Drawing for the job (mm, zero at the part's lowest x, y, z). A direction names the side the tool comes from. Coordinates: 2 decimals unless noted, no trailing zeros. Write each loop counter-clockwise with the first axis right and the second up, starting at its lowest first coordinate (ties: lowest second). Pieces come first, ordered by that corner, then holes. Notation, with made-up numbers: (-11, 83.5) - (32, 83.5) arc R20 cw to (32, 88.5) - close; hole circle Ø1 at (43, -1). An arc over 180 degrees is marked (long way). Write each question's results on one line, items separated by ' | '.
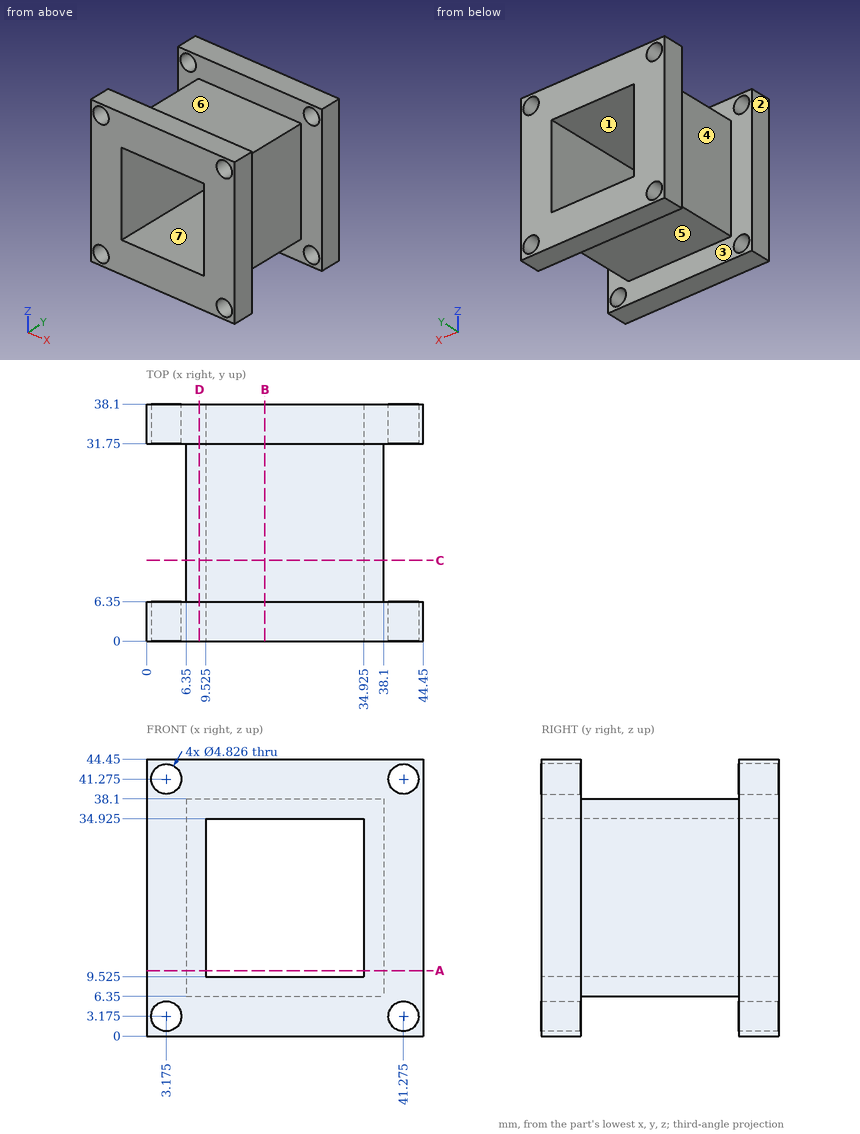
(1) Saw through at C-C on y = 13. Write the cut outline in (x, z) (3 decimals), then the cut area to 3 significant figures.
Return value:
outline: (6.35, 6.35) - (38.1, 6.35) - (38.1, 38.1) - (6.35, 38.1) - close; hole (9.525, 9.525) - (34.925, 9.525) - (34.925, 34.925) - (9.525, 34.925) - close | area: 363 mm^2
(2) Two-plate mould, pull along X, no slides. Class the marked faces 1, 2 and 3: released by +X, released by -X, zero draft, split by the parting line, or undercut.
Return value:
face 1: undercut | face 2: released by -X | face 3: zero draft
(3) Saw through at A-A on z = 10.5. Write the cut outline in (x, y) (3 decimals).
Return value:
outline: (0, 0) - (9.525, 0) - (9.525, 38.1) - (0, 38.1) - (0, 31.75) - (6.35, 31.75) - (6.35, 6.35) - (0, 6.35) - close; (34.925, 0) - (44.45, 0) - (44.45, 6.35) - (38.1, 6.35) - (38.1, 31.75) - (44.45, 31.75) - (44.45, 38.1) - (34.925, 38.1) - close
(4) Saw through at D-D on x = 8.5. Write the cut outline in (y, z).
Return value:
outline: (0, 0) - (6.35, 0) - (6.35, 6.35) - (31.75, 6.35) - (31.75, 0) - (38.1, 0) - (38.1, 44.45) - (31.75, 44.45) - (31.75, 38.1) - (6.35, 38.1) - (6.35, 44.45) - (0, 44.45) - close
(5) 3-axis set-ups, long thin cutter, end or side, ignore diameter. For the marked faces 4, 5, 6 and 7: which of +Z, -Z, +X, -X, +Y, -Y reach the whole face in a straight line?
Return value:
face 4: +Z, -Z, -X | face 5: -Z, +X, -X | face 6: +Z, +X, -X | face 7: +Y, -Y
(6) Flat gauge pins, fed straight in: P1, Ø4, axis at y = 31.5, z = 23, coming from the +X side; P2, Ø7.5, axis at y = 16, z = 20.5, coming from the -X side; P3, Ø12.5, axis at y = 19.5, z = 27, coming from the +X side; P4, Ø4, axis at x = 3.175, z = 41.275, coming from the -Y side. Where does each tip first touch, or does it go through?
Return value:
P1: stops at x = 44.45 | P2: stops at x = 6.35 | P3: stops at x = 38.1 | P4: passes through
(7) Saw through at B-B on x = 19. Write the cut outline in (y, z) (3 decimals).
Return value:
outline: (0, 0) - (6.35, 0) - (6.35, 6.35) - (31.75, 6.35) - (31.75, 0) - (38.1, 0) - (38.1, 9.525) - (0, 9.525) - close; (0, 34.925) - (38.1, 34.925) - (38.1, 44.45) - (31.75, 44.45) - (31.75, 38.1) - (6.35, 38.1) - (6.35, 44.45) - (0, 44.45) - close
(8) Wall check: line 1 (Z direction, x = 19, y = 36.5) (3 decimals); line 2 (Z direction, x = 27, y = 30) (3 decimals). Give the ranges that are in metal, low to high. Write a range as from..to.
Return value:
line 1: z = 0..9.525, 34.925..44.45 | line 2: z = 6.35..9.525, 34.925..38.1
